from build123d import *

# Parameters (mm, degrees)
SKETCH1_W           = 322
SKETCH1_H           = 322
SKETCH1_W_2         = 100
BOSS_EXTRUDE1_DEPTH = 55
SKETCH2_W           = 476
SKETCH2_H           = 358
BOSS_EXTRUDE2_DEPTH = 18


with BuildPart() as part:
    # Sketch1 → Boss-Extrude1 (new body)
    with BuildSketch(Plane.XY):
        Polygon((-18, -18), (340, -18), (458, -18), (458, 340), (340, 340), (-18, 340), align=None)
        with Locations((161, 161)):
            Rectangle(SKETCH1_W, SKETCH1_H, mode=Mode.SUBTRACT)
        with Locations((390, 161)):
            Rectangle(SKETCH1_W_2, SKETCH1_H, mode=Mode.SUBTRACT)
    extrude(amount=BOSS_EXTRUDE1_DEPTH)

    # Sketch2 → Boss-Extrude2 (add)
    with BuildSketch(Plane(origin=(0, 0, 0), x_dir=(-1, 0, 0), z_dir=(0, 0, -1))):
        with Locations((-220, 161)):
            Rectangle(SKETCH2_W, SKETCH2_H)
    extrude(amount=BOSS_EXTRUDE2_DEPTH)


solid = part.part
Can you work these out from the model? Positions are in its coordinate system, mm. A direction names the side the tool comes from. Coordinates: 2 decimals unless noted, no trailing zeros. Order: outer loops, then holes, each group sorted by start corner. A loop starts at its lowest first (then second) coordinate and runs counter-clockwise, first axis right, second up. Notation, with made-up numbers: (-0.5, -17) - (41.5, -17) arc R6 ccw to (41.5, -11) - close; hole circle Ø3 at (43, 65). An arc over 180 degrees is marked (long way). Answer as a JSON object with one key per item and string values. Group by question number.
Q1. Will this pin go through, and if not, where does the flat tip stop? P1, Ø10, axis at x = 283.5, y = 241.5, coming from the +Z side.
Q2. Imagine slicing it at A-A (z = 15). Please give me the cut outline in (x, y), and give its area (3 significant figures).
Q3. Imagine slicing it at B-B (y = 211). Please give me the cut outline in (x, z), and give its area (3 significant figures).
Q4. On a 3-axis mill with a long thin cutter (end or side, diameter ignored), from which of +Z, -Z, +X, -X, +Y, -Y can I reach the whole of each face in a straight line? I mean faces 1 (the face through (163, 163, 0)), 2 (the face through (458, 158, 19)). Say none if no direction works.
Q5. Imagine slicing it at C-C (x = 362). Please give me the cut outline in (y, z).
Q6. We'd pull the mould along X, two halves only. Please class faces 3 (the face through (-18, 158, 19)), 4 (the face through (159, 0, 27)), 5 (the face through (223, -18, 19)): +X half, -X half, draft (parallel to the pull), parting line (faces both ways), or undercut.
Q7. I need wall thicknesses on line 1 (X direction, y = 166.5, z = 25); line 2 (Y direction, x = 405.5, z = 11); line 3 (Z direction, x = 353, y = 187.5). Which ranges of each line are inside material? Lowest first, please. Write a range as from..to.
Determined:
{
 "1": {"P1": "stops at z = 0"},
 "2": {"outline": "(-18, -18) - (458, -18) - (458, 340) - (-18, 340) - close; hole (0, 0) - (322, 0) - (322, 322) - (0, 322) - close; hole (340, 0) - (440, 0) - (440, 322) - (340, 322) - close", "area": "34,500 mm2"},
 "3": {"outline": "(-18, -18) - (458, -18) - (458, 55) - (440, 55) - (440, 0) - (340, 0) - (340, 55) - (322, 55) - (322, 0) - (0, 0) - (0, 55) - (-18, 55) - close", "area": "11,500 mm2"},
 "4": {"face 1": "+Z", "face 2": "+Z, -Z, +X, +Y, -Y"},
 "5": {"outline": "(-18, -18) - (340, -18) - (340, 55) - (322, 55) - (322, 0) - (0, 0) - (0, 55) - (-18, 55) - close"},
 "6": {"face 3": "-X half", "face 4": "undercut", "face 5": "draft"},
 "7": {"line 1": "x = -18..0, 322..340, 440..458", "line 2": "y = -18..0, 322..340", "line 3": "z = -18..0"}
}
